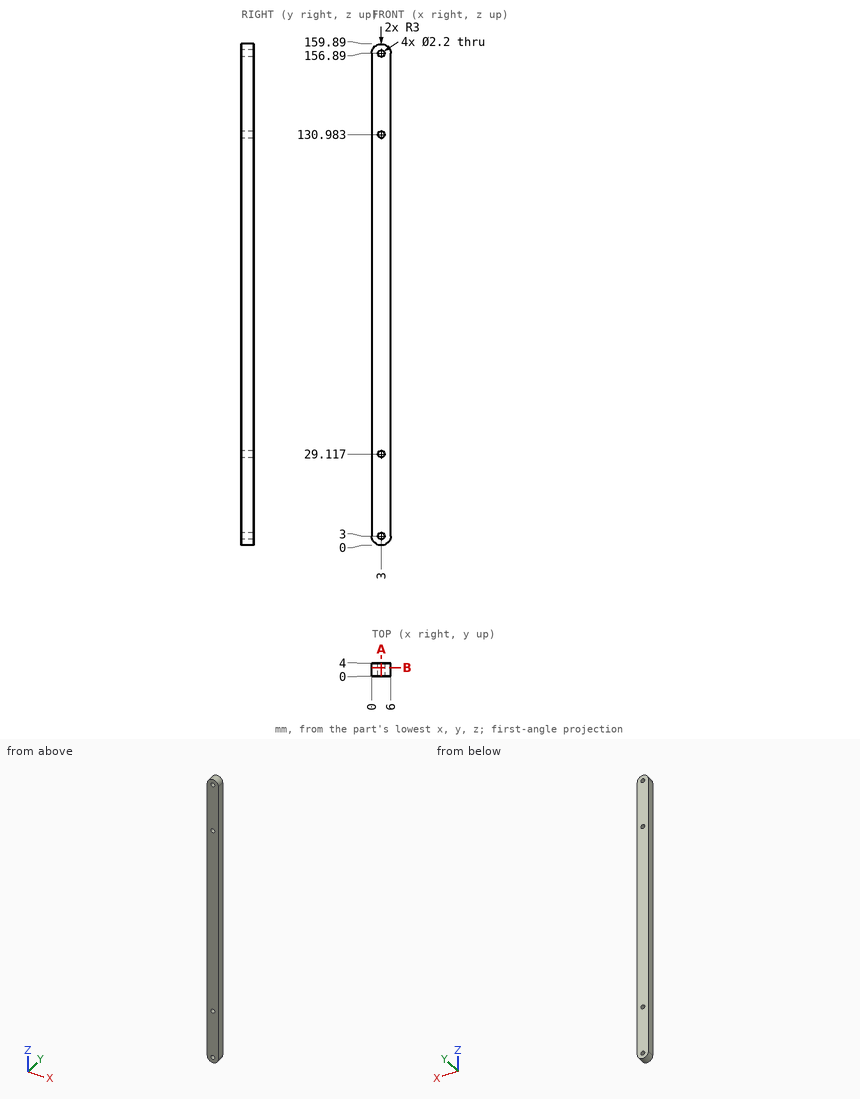
For this review, use the dimensioned drawing (mm, ordinates from the lowest corner) and the shaded views. Give positions to 0.01 mm unless a question says otherwise; leave off trailing zeros. Order: outer loops, then holes, each group sorted by start corner. A loop starts at its lowest first (then second) coordinate and runs counter-clockwise, first axis right, second up.
1. Add section B-B, the plane y = 2.65. State the section outline as (x, z) points, then the cut area to 3 significant figures.
Solution:
outline: (0, 3) arc R3 ccw to (6, 3) - (6, 156.89) arc R3 ccw to (0, 156.89) - close; hole circle Ø2.2 at (3, 3); hole circle Ø2.2 at (3, 29.12); hole circle Ø2.2 at (3, 130.98); hole circle Ø2.2 at (3, 156.89)
area: 936 mm2
2. Add section A-A, the plane x = 3. State the section outline as (y, z) points, then the cut area to 3 significant figures.
Solution:
outline: (0, 0) - (4, 0) - (4, 1.9) - (0, 1.9) - close; (0, 4.1) - (4, 4.1) - (4, 28.02) - (0, 28.02) - close; (0, 30.22) - (4, 30.22) - (4, 129.88) - (0, 129.88) - close; (0, 132.08) - (4, 132.08) - (4, 155.79) - (0, 155.79) - close; (0, 157.99) - (4, 157.99) - (4, 159.89) - (0, 159.89) - close
area: 604 mm2
3. For pin 1 Ø1 at (x, y) = (1.5, 1.5) entering from +Z, flat-tipped, find the tip position at first contact; note if it passes through.
Solution:
pin 1: stops at z = 159.72
4. To check wall thickness, follow L1, parallel to Z at x = 3, y = 1.5; L2, parallel to Z at x = 2.05, y = 0.25; L3, parallel to X at y = 1.95, z = 156.89. State the ranges of each line that lie inside material, in increasing order.
Solution:
L1: z = 0 to 1.9, 4.1 to 28.02, 30.22 to 129.88, 132.08 to 155.79, 157.99 to 159.89
L2: z = 0.15 to 2.45, 3.55 to 28.56, 29.67 to 130.43, 131.54 to 156.34, 157.44 to 159.74
L3: x = 0 to 1.9, 4.1 to 6
